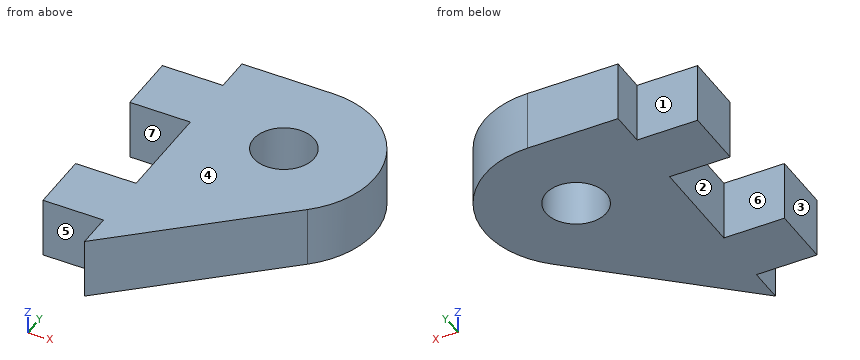
from build123d import *

# Parameters (mm, degrees)
SKETCH1_R           = 1.5
BOSS_EXTRUDE1_DEPTH = 1.5
SKETCH2_W           = 3
SKETCH2_H           = 3
BOSS_EXTRUDE2_DEPTH = 3


with BuildPart() as part:
    # Sketch1 → Boss-Extrude1 (new body, symmetric)
    with BuildSketch(Plane.XY):
        with BuildLine():
            Line((0, 0), (0, 10))
            Line((0, 10), (0, 14.5))
            Line((0, 14.5), (4.5, 14.5))
            ThreePointArc((4.5, 14.5), (8.707488868, 11.595944054), (7.484407484, 6.632016632))
            Line((7.484407484, 6.632016632), (0, 0))
        make_face()
        with Locations((4.5, 10)):
            Circle(SKETCH1_R, mode=Mode.SUBTRACT)
    extrude(amount=BOSS_EXTRUDE1_DEPTH, both=True)

    # Sketch2 → Boss-Extrude2 (add)
    with BuildSketch(Plane.ZY):
        with Locations((0, 11.25)):
            Rectangle(SKETCH2_W, SKETCH2_H)
        with Locations((0, 3.25)):
            Rectangle(SKETCH2_W, SKETCH2_H)
    extrude(amount=BOSS_EXTRUDE2_DEPTH)


solid = part.part
Geometry check sheet. Reference: the model listing, model coordinates, mm. Face numbers are marked on the shaded views. A direction names the side the tool comes from. Round coordinates to 2 decimals unless told otherwise and drop trailing zeros. Loops run counter-clockwise (first coordinate to the right, second up) from the corner with the lowest first, then second, coordinate; pieces in that order, holes last.
Item 1: Cross-section at A-A on y = 10. Record the boundary of the cut face in (x, z).
Item 2: Mould release check, pull along Y, two halves, no side actions. Record for the marked faces 4, 5, 6 and 7: pulls with the +Y half, pulls with the -Y half, needs draft (parallel to the pull), parting line crosses it, or undercut.
Item 3: Thickness scan on line 1 (X direction, y = 10.5, z = 1.3); line 2 (X direction, y = 9.25, z = -0.1); line 3 (Y direction, x = 4.5, z = 0.7). Record the ranges inside material, lowest first.
Item 4: Cross-section at C-C on x = -2.5. Record the boundary of the cut face in (y, z), then the cut area to 3 significant figures.
Item 5: Cross-section at D-D on x = 7. Record the boundary of the cut face in (y, z), then the cut area to 3 significant figures.
Item 6: Cross-section at B-B on z = 0.75. Record the boundary of the cut face in (x, y), then the cut area to 3 significant figures.
Item 7: Access from +Z, -Z, +X, -X, +Y, -Y to the whole of each face (thin tool, end or side, straight path). Record for the marked faces 1, 2 and 3.
Item 8: Gauge pin test, flat ends, axial feed: pin 1 (0.9 mm diameter, centred on x = -1, z = -0.5, fed in from -Y); pin 2 (0.9 mm diameter, centred on x = -1.5, z = 0.5, fed in from +Y); pin 3 (1.5 mm diameter, centred on y = 11, z = 0, fed in from +X). Record the tip position at first contact, or that the pin passes through.
Answer sheet:
1. outline: (-3, -1.5) - (3, -1.5) - (3, 1.5) - (-3, 1.5) - close; (6, -1.5) - (9, -1.5) - (9, 1.5) - (6, 1.5) - close
2. face 4: needs draft
2. face 5: pulls with the -Y half
2. face 6: undercut
2. face 7: undercut
3. line 1: x = -3 to 3.09, 5.91 to 8.97
3. line 2: x = 0 to 3.2, 5.8 to 8.94
3. line 3: y = 3.99 to 8.5, 11.5 to 14.5
4. outline: (1.75, -1.5) - (4.75, -1.5) - (4.75, 1.5) - (1.75, 1.5) - close; (9.75, -1.5) - (12.75, -1.5) - (12.75, 1.5) - (9.75, 1.5) - close
4. area: 18.0 mm2
5. outline: (6.2, -1.5) - (13.74, -1.5) - (13.74, 1.5) - (6.2, 1.5) - close
5. area: 22.6 mm2
6. outline: (-3, 1.75) - (0, 1.75) - (0, 0) - (7.48, 6.63) arc R4.5 ccw to (4.5, 14.5) - (0, 14.5) - (0, 12.75) - (-3, 12.75) - (-3, 9.75) - (0, 9.75) - (0, 4.75) - (-3, 4.75) - close; hole circle Ø3 at (4.5, 10)
6. area: 101 mm2
7. face 1: +Z, -Z, -X, +Y
7. face 2: +Z, -Z, -X
7. face 3: +Z, -Z, -X, +Y, -Y
8. pin 1: stops at y = 1.75
8. pin 2: stops at y = 12.75
8. pin 3: stops at x = 8.99
